from build123d import *

# Parameters (mm, degrees)
F0_W     = 16.5
F0_H     = 10
F0_W_2   = 11
F0_H_2   = 3
F1_DEPTH = 6
F2_R     = 1.5
F0_W_3   = 5.5
F0_H_3   = 1.5
F3_DEPTH = 0.6


with BuildPart() as f1:
    # F0 (on Top) → F1 (new body)
    with BuildSketch(Plane.XY):
        with Locations((0, 0.571325)):
            Rectangle(F0_W, F0_H)
        Rectangle(F0_W_2, F0_H_2, mode=Mode.SUBTRACT)
    extrude(amount=F1_DEPTH)

    # F2
    f2_edges = [f1.edges().sort_by_distance(p)[0] for p in [
        (-8.25, 5.571325, 3),
        (8.25, 5.571325, 3),
        (8.25, -4.428675, 3),
        (-8.25, -4.428675, 3),
    ]]
    fillet(f2_edges, radius=F2_R)

    # F0 (on Top) → F3 (join)
    with BuildSketch(Plane.XY):
        Rectangle(F0_W_2, F0_H_2)
        Rectangle(F0_W_3, F0_H_3, mode=Mode.SUBTRACT)
    extrude(amount=F3_DEPTH)


solid = f1.part
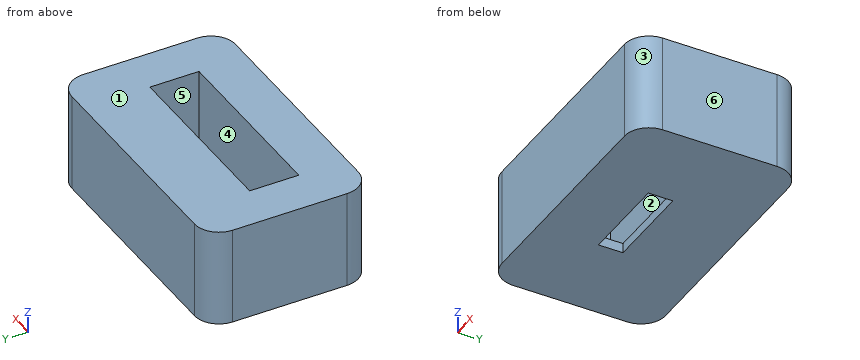
Part model, mm, in its own coordinate system. Face numbers are marked on the shaded views. A direction names the side the tool comes from. Give positions to 0.01 mm unless a question says otherwise; leave off trailing zeros. Order: outer loops, then holes, each group sorted by start corner. A loop starts at its lowest first (then second) coordinate and runs counter-clockwise, first axis right, second up. Notation, with made-up numbers: (83.25, -12.75) - (102.25, -12.75) arc R13 ccw to (102.25, 9.25) - close; hole circle Ø7 at (-9, 70.25). An arc over 180 degrees is marked (long way). One line per question, with ' | ' between items.
1. Band-saw the part on A-A on x = -1.5. List the corners of the cut face in (y, z).
Filled in:
outline: (-4.43, 0) - (-0.75, 0) - (-0.75, 0.6) - (-1.5, 0.6) - (-1.5, 6) - (-4.43, 6) - close; (0.75, 0) - (5.57, 0) - (5.57, 6) - (1.5, 6) - (1.5, 0.6) - (0.75, 0.6) - close
2. Drill centre lines: probe 1 along Y at (x, z) = (-1.25, 3); probe 2 along X at (y, z) = (1.25, 0.95); probe 3 along Z at (x, y) = (0.5, -1.25). Where is each one in solid material? Low to high.
Filled in:
probe 1: -4.43 to -1.5, 1.5 to 5.57 | probe 2: -8.25 to -5.5, 5.5 to 8.25 | probe 3: 0 to 0.6
3. Band-saw the part on C-C on x = -4.5. List the corners of the cut face in (y, z).
Filled in:
outline: (-4.43, 0) - (5.57, 0) - (5.57, 6) - (1.5, 6) - (1.5, 0.6) - (-1.5, 0.6) - (-1.5, 6) - (-4.43, 6) - close
4. Which spindle directions (+Z, -Z, +X, -X, +Y, -Y) get a long thin tool onto all of the face, cutting with end or side? Do the marked faces 5 and 6. Say none if no direction does.
Filled in:
face 5: +Z | face 6: +Z, -Z, +X, +Y, -Y
5. Pull direction X, two halves, no side cores. Call the marked faces 1, 2, 3 and 4: +X half, -X half, draft (parallel to the pull), parting line (faces both ways), or undercut.
Filled in:
face 1: draft | face 2: undercut | face 3: +X half | face 4: undercut
6. Band-saw the part on D-D on z = 0.4. List the corners of the cut face in (x, y), then the cut area to 3 significant figures.
Filled in:
outline: (-8.25, -2.93) arc R1.5 ccw to (-6.75, -4.43) - (6.75, -4.43) arc R1.5 ccw to (8.25, -2.93) - (8.25, 4.07) arc R1.5 ccw to (6.75, 5.57) - (-6.75, 5.57) arc R1.5 ccw to (-8.25, 4.07) - close; hole (-2.75, -0.75) - (2.75, -0.75) - (2.75, 0.75) - (-2.75, 0.75) - close | area: 155 mm²
7. Band-saw the part on B-B on z = 5.6. List the corners of the cut face in (x, y).
Filled in:
outline: (-8.25, -2.93) arc R1.5 ccw to (-6.75, -4.43) - (6.75, -4.43) arc R1.5 ccw to (8.25, -2.93) - (8.25, 4.07) arc R1.5 ccw to (6.75, 5.57) - (-6.75, 5.57) arc R1.5 ccw to (-8.25, 4.07) - close; hole (-5.5, -1.5) - (5.5, -1.5) - (5.5, 1.5) - (-5.5, 1.5) - close
